```python
from build123d import *

# Parameters (mm, degrees)
F1_DEPTH = 225
F2_W     = 3
F2_H     = 340
F3_DEPTH = 25
F5_DEPTH = 12.001


with BuildPart() as f1:
    # F0 (on Top) → F1 (new body, symmetric)
    with BuildSketch(Plane.XY):
        with BuildLine():
            ThreePointArc((20, 18), (19.414214, 19.414214), (18, 20))
            Line((18, 20), (-18, 20))
            ThreePointArc((-18, 20), (-19.414214, 19.414214), (-20, 18))
            Line((-20, 18), (-20, -18))
            ThreePointArc((-20, -18), (-19.414214, -19.414214), (-18, -20))
            Line((-18, -20), (18, -20))
            ThreePointArc((18, -20), (19.414214, -19.414214), (20, -18))
            Line((20, -18), (20, 18))
        make_face()
        with BuildLine():
            Line((-15, 17), (15, 17))
            ThreePointArc((15, 17), (16.414214, 16.414214), (17, 15))
            Line((17, 15), (17, -15))
            ThreePointArc((17, -15), (16.414214, -16.414214), (15, -17))
            Line((15, -17), (-15, -17))
            ThreePointArc((-15, -17), (-16.414214, -16.414214), (-17, -15))
            Line((-17, -15), (-17, 15))
            ThreePointArc((-17, 15), (-16.414214, 16.414214), (-15, 17))
        make_face(mode=Mode.SUBTRACT)
    extrude(amount=F1_DEPTH, both=True)

    # F2 (on face) → F3 (join)
    with BuildSketch(Plane.YZ.offset(20)):
        with Locations((9.5, 55)):
            Rectangle(F2_W, F2_H)
    extrude(amount=F3_DEPTH)

    # F4 (on face) → F5 (cut, through all)
    with BuildSketch(Plane.XZ.offset(-8)):
        Polygon((45, 225), (20, 225), (45, 200), align=None)
        Polygon((45, -115), (45, -90), (20, -115), align=None)
    extrude(amount=-F5_DEPTH, mode=Mode.SUBTRACT)


solid = f1.part
```
Geometry check sheet. Reference: the model listing, model coordinates, mm. A direction names the side the tool comes from. Give positions to 0.01 mm unless a question says otherwise; leave off trailing zeros. Order: outer loops, then holes, each group sorted by start corner. A loop starts at its lowest first (then second) coordinate and runs counter-clockwise, first axis right, second up.
1. Section check A-A, the plane x = -3. Enter the section's corners in (y, z).
2. Section check C-C, the plane x = 39.5. Enter the section's corners in (y, z).
3. Thickness scan on L1, parallel to X at y = -3, z = 200; L2, parallel to X at y = 9, z = 50.5. Record the ranges inside material, lowest first.
4. Gauge pin test, flat ends, axial feed: pin 1 Ø20 at (x, z) = (28.5, 88.5) entering from -Y; pin 2 Ø8 at (x, y) = (8, -12) entering from +Z; pin 3 Ø12.5 at (x, z) = (34.5, 67) entering from +Y; pin 4 Ø4 at (x, z) = (25.5, -52.5) entering from -Y. Record the tip position at first contact, or that the pin passes through.
5. Release check for a two-part mould opening along Y. For faces 1 (the face through (-17, 0, 3)), 2 (the face through (0, 17, 3)), 3 (the face through (32, 9, 213)), 4 (the face through (32, 11, 53)) record: pulls with the +Y half, pulls with the -Y half, needs draft (parallel to the pull), parting line crosses it, or undercut.
6. Access from +Z, -Z, +X, -X, +Y, -Y to the whole of each face (thin tool, end or side, straight path). Record for faces 5 (the face through (17, 0, 3)), 6 (the face through (0, 20, 3)), 7 (the face through (32, 8, 53)).
7. Section check D-D, the plane z = -190. Enter the section's corners in (x, y).
8. Section check B-B, the plane z = -18. Enter the section's corners in (x, y), and give its area (3 significant figures).
Values follow:
1. outline: (-20, -225) - (-17, -225) - (-17, 225) - (-20, 225) - close; (17, -225) - (20, -225) - (20, 225) - (17, 225) - close
2. outline: (8, -95.5) - (11, -95.5) - (11, 205.5) - (8, 205.5) - close
3. L1: x = -20 to -17, 17 to 20
3. L2: x = -20 to -17, 17 to 45
4. pin 1: stops at y = -19.94
4. pin 2: passes through
4. pin 3: stops at y = 11
4. pin 4: stops at y = 8
5. face 1: undercut
5. face 2: undercut
5. face 3: needs draft
5. face 4: pulls with the +Y half
6. face 5: +Z, -Z
6. face 6: +Z, -Z, +X, -X, +Y
6. face 7: +Z, -Z, +X, -Y
7. outline: (-20, -18) arc R2 ccw to (-18, -20) - (18, -20) arc R2 ccw to (20, -18) - (20, 18) arc R2 ccw to (18, 20) - (-18, 20) arc R2 ccw to (-20, 18) - close; hole (-17, -15) arc R2 ccw to (-15, -17) - (15, -17) arc R2 ccw to (17, -15) - (17, 15) arc R2 ccw to (15, 17) - (-15, 17) arc R2 ccw to (-17, 15) - close
8. outline: (-20, -18) arc R2 ccw to (-18, -20) - (18, -20) arc R2 ccw to (20, -18) - (20, 8) - (45, 8) - (45, 11) - (20, 11) - (20, 18) arc R2 ccw to (18, 20) - (-18, 20) arc R2 ccw to (-20, 18) - close; hole (-17, -15) arc R2 ccw to (-15, -17) - (15, -17) arc R2 ccw to (17, -15) - (17, 15) arc R2 ccw to (15, 17) - (-15, 17) arc R2 ccw to (-17, 15) - close
8. area: 519 mm2
